```python
from build123d import *

# Parameters (mm, degrees)
F0_W      = 106.9598533213
F0_H      = 19.4777743891
F1_DEPTH  = 55.88
F3_DEPTH  = 25.4
F4_W      = 57.0900328457
F4_H      = 35.8569398522
F5_DEPTH  = 25.4
F7_DEPTH  = 35.56
F8_W      = 32.9107241705
F8_H      = 18.7523802742
F9_DEPTH  = 10.16
F11_DEPTH = 20.32


with BuildPart() as f1:
    # F0 (on Front) → F1 (new body)
    with BuildSketch(Plane.XZ):
        with Locations((-7.975814864, 2.0988979377)):
            Rectangle(F0_W, F0_H)
    extrude(amount=F1_DEPTH)

    # F2 (on face) → F3 (cut)
    with BuildSketch(Plane.XY.offset(11.8377851322)):
        Polygon((45.5041117966, -27.94), (4.7015314922, -55.88), (45.5041117966, -55.88), align=None)
        Polygon((-61.4557415247, -55.88), (-28.377102688, -55.88), (-61.4557415247, -24.0953527391), align=None)
    extrude(amount=-F3_DEPTH, mode=Mode.SUBTRACT)

    # F4 (on Front) → F5 (join)
    with BuildSketch(Plane.XZ):
        with Locations((-5.2052680403, 29.6829007566)):
            Rectangle(F4_W, F4_H)
    extrude(amount=F5_DEPTH)

    # F6 (on face) → F7 (cut)
    with BuildSketch(Plane.XY.offset(47.6113706827)):
        Polygon((23.3397483826, -10.4944910854), (3.6940614227, -25.4), (23.3397483826, -25.4), align=None)
        Polygon((-33.7502844632, -25.4), (-17.4628347158, -25.4), (-33.7502844632, -10.4944910854), align=None)
    extrude(amount=-F7_DEPTH, mode=Mode.SUBTRACT)

    # F8 (on face) → F9 (join)
    with BuildSketch(Plane.XZ.offset(55.88)):
        with Locations((-11.7538305931, 21.2139752693)):
            Rectangle(F8_W, F8_H)
    extrude(amount=-F9_DEPTH)

    # F10 (on face) → F11 (cut)
    with BuildSketch(Plane.XZ.offset(55.88)):
        with BuildLine():
            Line((-3.0823028615, 13.2553465664), (-10.0014163181, 13.2553465664))
            Line((-10.0014163181, 13.2553465664), (-10.0014163181, 6.3362331098))
            ThreePointArc((-10.0014163181, 6.3362331098), (-5.1088642731, 8.3627945214), (-3.0823028615, 13.2553465664))
        make_face()
        with BuildLine():
            Line((-10.0014163181, 6.3362331098), (-10.0014163181, 13.2553465664))
            Line((-10.0014163181, 13.2553465664), (-16.8943863629, 13.856258363))
            ThreePointArc((-16.8943863629, 13.856258363), (-15.1020000065, 8.5800736264), (-10.0014163181, 6.3362331098))
        make_face()
        with BuildLine():
            Line((-16.8943863629, 13.856258363), (-10.0014163181, 13.2553465664))
            Line((-10.0014163181, 13.2553465664), (-9.4005045216, 20.1483166113))
            ThreePointArc((-9.4005045216, 20.1483166113), (-14.4505733731, 18.5543212339), (-16.8943863629, 13.856258363))
        make_face()
        with BuildLine():
            Line((-9.4005045216, 20.1483166113), (-10.0014163181, 13.2553465664))
            Line((-10.0014163181, 13.2553465664), (-3.0823028615, 13.2553465664))
            ThreePointArc((-3.0823028615, 13.2553465664), (-4.9008326298, 17.9306195065), (-9.4005045216, 20.1483166113))
        make_face()
    extrude(amount=-F11_DEPTH, mode=Mode.SUBTRACT)


solid = f1.part
```
CAD build for the part. Positions are in the model's coordinates, mm. A direction names the side the tool comes from. Round coordinates to 2 decimals unless told otherwise and drop trailing zeros. Write each loop counter-clockwise with the first axis right and the second up, starting at its lowest first coordinate (ties: lowest second). Pieces come first, ordered by that corner, then holes. Notation, with made-up numbers: (-34.75, 36) -> (4.25, 36) arc R12 ccw to (4.25, 53) -> close; hole circle Ø1 at (-27.5, -14.5). An arc over 180 degrees is marked (long way). Answer in a Markdown table with one row per item. Add a question column.
Item 1: Drop flat-ended pins along their axis: pin 1 Ø3 at (y, z) = (-51.5, 16.5) entering from +X; pin 2 Ø7.5 at (y, z) = (-15, 30.5) entering from +X; pin 3 Ø5 at (x, y) = (-4.5, -50) entering from +Z. Give the stop position or say it passes through.
Item 2: Drill centre lines: line 1 (Y direction, x = -5, z = 23.5); line 2 (X direction, y = -4, z = 25); line 3 (Z direction, x = -45, y = -5). Where is each one in solid material? Low to high. Write a range as from..to.
Item 3: Saw through at A-A, the plane y = -50.5. Write the cut outline in (x, z).
Item 4: Saw through at D-D, the plane y = -8. Write the cut outline in (x, z).
Item 5: Mould opens along Y. For faces 1 (the face through (45.504, -14, 2)), 2 (the face through (-10, -35.56, 10)), 3 (the face through (-5, -25.4, 30)) say: pulls with the +Y half, pulls with the -Y half, needs draft (parallel to the pull), parting line crosses it, or undercut.
Item 6: Saw through at B-B, the plane x = 10. Write the cut outline in (y, z).
Item 7: Which spindle directions (+Z, -Z, +X, -X, +Y, -Y) get a long thin tool onto all of the face, cutting with end or side? Do faces 4 (the face through (-28.209, -51, 21)), 5 (the face through (-12, -51, 30.59)), 6 (the face through (23.34, -4, 29)), 7 (the face through (-33.75, -4, 29)), 8 (the face through (-25.493, -18.052, 30.08)). Say none if no direction does.
Item 8: Saw through at C-C, the plane z = 44.5. Write the cut outline in (x, y), then the cut area to 3 significant figures.
Findings below:
| question | item | result |
|---|---|---|
| 1 | pin 1 | stops at x = 4.7 |
| 1 | pin 2 | stops at x = 22.34 |
| 1 | pin 3 | stops at z = 30.59 |
| 2 | line 1 | y = -55.88..-45.72, -25.4..0 |
| 2 | line 2 | x = -33.75..23.34 |
| 2 | line 3 | z = -7.64..11.84 |
| 3 | outline | (-33.98, -7.64) -> (12.56, -7.64) -> (12.56, 11.84) -> (4.7, 11.84) -> (4.7, 30.59) -> (-28.21, 30.59) -> (-28.21, 11.84) -> (-33.98, 11.84) -> close; hole circle Ø13.84 at (-10, 13.26) |
| 4 | outline | (-61.46, -7.64) -> (45.5, -7.64) -> (45.5, 11.84) -> (23.34, 11.84) -> (23.34, 47.61) -> (-33.75, 47.61) -> (-33.75, 11.84) -> (-61.46, 11.84) -> close |
| 5 | face 1 | needs draft |
| 5 | face 2 | pulls with the -Y half |
| 5 | face 3 | undercut |
| 6 | outline | (-52.25, -7.64) -> (0, -7.64) -> (0, 47.61) -> (-20.62, 47.61) -> (-20.62, 12.05) -> (-25.4, 12.05) -> (-25.4, 11.84) -> (-52.25, 11.84) -> close |
| 7 | face 4 | +Z, -X, -Y |
| 7 | face 5 | +Z, +X, -X, -Y |
| 7 | face 6 | +Z, +X, +Y, -Y |
| 7 | face 7 | +Z, -X, +Y, -Y |
| 7 | face 8 | +Z, -X |
| 8 | outline | (-33.75, -10.49) -> (-17.46, -25.4) -> (3.69, -25.4) -> (23.34, -10.49) -> (23.34, 0) -> (-33.75, 0) -> close |
| 8 | area | 1,180 mm^2 |
